from build123d import *

# Parameters (mm, degrees)
BOSS_EXTRUDE1_DEPTH      = 60
BOSS_EXTRUDE1_DEPTH_BACK = 60
SKETCH1_W                = 400
SKETCH1_H                = 50
BOSS_EXTRUDE2_DEPTH      = 60
BOSS_EXTRUDE2_DEPTH_BACK = 60
SKETCH2_R                = 35
CUT_EXTRUDE1_DEPTH       = 60
CUT_EXTRUDE1_DEPTH_BACK  = 60
SKETCH3_R                = 10
CUT_EXTRUDE2_DEPTH       = 60
CUT_EXTRUDE2_DEPTH_BACK  = 60
SKETCH4_W                = 200
SKETCH4_H                = 25


with BuildPart() as part:
    # Sketch1 → Boss-Extrude1 (new, two sides: drawn at the far end of the back side and taken through both)
    with BuildSketch(Plane(origin=(0, 0, 0), x_dir=(1, 0, 0), z_dir=(0, 1, 0)).offset(-BOSS_EXTRUDE1_DEPTH_BACK)):
        with Locations((200, 0)):
            Rectangle(SKETCH1_W, SKETCH1_H)
    extrude(amount=BOSS_EXTRUDE1_DEPTH + BOSS_EXTRUDE1_DEPTH_BACK)

    # Sketch2 → Boss-Extrude2 (add, two sides: drawn at the far end of the back side and taken through both)
    with BuildSketch(Plane(origin=(0, 0, 0), x_dir=(1, 0, 0), z_dir=(0, 1, 0)).offset(-BOSS_EXTRUDE2_DEPTH_BACK)):
        Circle(SKETCH2_R)
        with Locations((400, 0)):
            Circle(SKETCH2_R)
    extrude(amount=BOSS_EXTRUDE2_DEPTH + BOSS_EXTRUDE2_DEPTH_BACK)

    # Sketch3 → Cut-Extrude1 (cut, two sides: drawn at the far end of the back side and taken through both)
    with BuildSketch(Plane(origin=(0, 0, 0), x_dir=(1, 0, 0), z_dir=(0, 1, 0)).offset(-CUT_EXTRUDE1_DEPTH_BACK)):
        with Locations(Location((0, 0, 0), (0, 0, 270))):
            Circle(SKETCH3_R)
        with Locations(Location((400, 0, 0), (0, 0, 270))):
            Circle(SKETCH3_R)
    extrude(amount=CUT_EXTRUDE1_DEPTH + CUT_EXTRUDE1_DEPTH_BACK, mode=Mode.SUBTRACT)

    # Sketch4 → Cut-Extrude2 (cut, two sides: drawn at the far end of the back side and taken through both)
    with BuildSketch(Plane(origin=(0, 0, 0), x_dir=(1, 0, 0), z_dir=(0, 1, 0)).offset(-CUT_EXTRUDE2_DEPTH_BACK)):
        with Locations((200, 0)):
            Rectangle(SKETCH4_W, SKETCH4_H)
    extrude(amount=CUT_EXTRUDE2_DEPTH + CUT_EXTRUDE2_DEPTH_BACK, mode=Mode.SUBTRACT)


solid = part.part
Input: part model. Units: mm. Frame: model coordinates. A direction names the side the tool comes from. Give positions to 0.01 mm unless a question says otherwise; leave off trailing zeros. Order: outer loops, then holes, each group sorted by start corner. A loop starts at its lowest first (then second) coordinate and runs counter-clockwise, first axis right, second up.
Q1. Draft query along Z for faces 1 (the cylindrical face through (-34.98, -0.84, -1.15)), 2 (the flat face through (197, 60, -16)), 3 (the flat face through (199, -1, 12.5)). Return one class per face: +Z half, -Z half, draft (parallel to the pull), parting line (faces both ways), or undercut.
Checked values:
face 1: parting line
face 2: draft
face 3: undercut
Q2. Contact query for flat-ended pins moving along their axis: pin 1 Ø7.5 at (y, z) = (-27, -5.5) entering from +X; pin 2 Ø2 at (y, z) = (-15, 22) entering from +X; pin 3 Ø2 at (y, z) = (-31, 16.5) entering from -X; pin 4 Ø18 at (x, z) = (400, 0) entering from +Y. Output: stop coordinate, or through.
Checked values:
pin 1: stops at x = 434.96
pin 2: stops at x = 428
pin 3: stops at x = -31.38
pin 4: passes through
Q3. Section B-B on x = 400. Output: boundary loops of the cut face in (y, z), and give its area (3 significant figures).
Checked values:
outline: (-60, -35) - (60, -35) - (60, -10) - (-60, -10) - close; (-60, 10) - (60, 10) - (60, 35) - (-60, 35) - close
area: 6,000 mm2
Q4. Section A-A on y = 36. Output: boundary loops of the cut face in (x, z).
Checked values:
outline: (24.49, -25) - (375.51, -25) arc R35 ccw (long way) to (375.51, 25) - (24.49, 25) arc R35 ccw (long way) to start; hole circle Ø20 at (0, 0); hole (100, -12.5) - (300, -12.5) - (300, 12.5) - (100, 12.5) - close; hole circle Ø20 at (400, 0)
Q5. Ray query, probe 1 along X at (y, z) = (14, 0); probe 2 along Z at (x, y) = (254, 4); probe 3 along X at (y, z) = (8, 4). Return the intervals inside material, ascending.
Checked values:
probe 1: x = -35 to -10, 10 to 100, 300 to 390, 410 to 435
probe 2: z = -25 to -12.5, 12.5 to 25
probe 3: x = -34.77 to -9.17, 9.17 to 100, 300 to 390.83, 409.17 to 434.77
Q6. Section C-C on z = 0. Output: boundary loops of the cut face in (x, y).
Checked values:
outline: (-35, -60) - (-10, -60) - (-10, 60) - (-35, 60) - close; (10, -60) - (100, -60) - (100, 60) - (10, 60) - close; (300, -60) - (390, -60) - (390, 60) - (300, 60) - close; (410, -60) - (435, -60) - (435, 60) - (410, 60) - close
Q7. Section D-D on x = 78. Output: boundary loops of the cut face in (y, z).
Checked values:
outline: (-60, -25) - (60, -25) - (60, 25) - (-60, 25) - close
Q8. Set-up query: faces 4 (the flat face through (198, -1, -25)), 5 (the flat face through (300, -1, 0)), 6 (the flat face through (198, -1, 25)), 7 (the flat face through (197, -60, -16)). Return all of +Z, -Z, +X, -X, +Y, -Y with unobstructed straight access to the full face (end or side cutting, diameter ignored); none if empty.
Checked values:
face 4: -Z, +Y, -Y
face 5: +Y, -Y
face 6: +Z, +Y, -Y
face 7: +Z, -Z, +X, -X, -Y
